Build history of the part. All positions in model axes, mm. A direction names the side the tool comes from. Give positions to 0.01 mm unless a question says otherwise; leave off trailing zeros. Write each loop counter-clockwise with the first axis right and the second up, starting at its lowest first coordinate (ties: lowest second). Pieces come first, ordered by that corner, then holes. Notation, with made-up numbers: (-9.75, 64) - (28.25, 64) arc R33 ccw to (28.25, 93) - close; hole circle Ø11 at (-37.75, 0.25). An arc over 180 degrees is marked (long way). Use one line per item in the form item = value. Start each with the question number.
from build123d import *

# Parameters (mm, degrees)
F1_DEPTH = 20
F2_W     = 5
F2_H     = 10
F3_DEPTH = 29.868809509


with BuildPart() as f1:
    # F0 (on Top) → F1 (new body)
    with BuildSketch(Plane.XY):
        with BuildLine():
            ThreePointArc((-34.9428019347, -9.9991262455), (-27.7864355102, -7.117650768), (-24.8106114437, 0))
            ThreePointArc((-24.8106114437, 0), (-27.6929606757, 7.0241759335), (-34.6784209527, 9.9991262455))
            Line((-34.6784209527, 9.9991262455), (-34.9428019347, 9.9991262455))
            Line((-34.9428019347, 9.9991262455), (-34.9428019347, 4.998252262))
            ThreePointArc((-34.9428019347, 4.998252262), (-31.3221269916, 3.581965414), (-29.8106114437, 0))
            ThreePointArc((-29.8106114437, 0), (-31.3221269916, -3.581965414), (-34.9428019347, -4.998252262))
            Line((-34.9428019347, -4.998252262), (-34.9428019347, -9.9991262455))
        make_face()
        with BuildLine():
            ThreePointArc((-34.6784209527, 9.9991262455), (-27.6929606757, 7.0241759335), (-24.8106114437, 0))
            ThreePointArc((-24.8106114437, 0), (-27.7864355102, -7.117650768), (-34.9428019347, -9.9991262455))
            Line((-34.9428019347, -9.9991262455), (-34.9428019347, -10.0008737545))
            Line((-34.9428019347, -10.0008737545), (-14.9428019347, -10.0008737545))
            Line((-14.9428019347, -10.0008737545), (-14.9428019347, 9.9991262455))
            Line((-14.9428019347, 9.9991262455), (-34.6784209527, 9.9991262455))
        make_face()
        with BuildLine():
            Line((-34.9428019347, 9.9991262455), (-34.6784209527, 9.9991262455))
            ThreePointArc((-34.6784209527, 9.9991262455), (-34.8106114437, 10), (-34.9428019347, 9.9991262455))
        make_face()
        with BuildLine():
            ThreePointArc((-34.9428019347, 9.9991262455), (-44.8106114437, 0), (-34.9428019347, -9.9991262455))
            Line((-34.9428019347, -9.9991262455), (-34.9428019347, -4.998252262))
            ThreePointArc((-34.9428019347, -4.998252262), (-39.8106114437, 0), (-34.9428019347, 4.998252262))
            Line((-34.9428019347, 4.998252262), (-34.9428019347, 9.9991262455))
        make_face()
    extrude(amount=F1_DEPTH)

    # F2 (on face) → F3 (cut, through all)
    with BuildSketch(Plane.YZ.offset(-14.9428019347)):
        with Locations((-0.0008737545, 15)):
            Rectangle(F2_W, F2_H)
    extrude(amount=-F3_DEPTH, mode=Mode.SUBTRACT)


solid = f1.part
(1) Which spindle directions (+Z, -Z, +X, -X, +Y, -Y) get a long thin tool onto all of the face, cutting with end or side? Do faces 4 (the flat face through (-27, 6, 20)), 5 (the flat face through (-23, -2.501, 15)). Say none if no direction does.
(2) Two-plate mould, pull along Y, no slides. Class faces 1 (the flat face through (-27, 0, 0)), 2 (the flat face through (-25, 9.999, 10)), 3 (the flat face through (-42, 2.499, 15)): +Y half, -Y half, draft (parallel to the pull), parting line (faces both ways), or undercut.
(3) Wall check: line 1 (Y direction, x = -22.5, z = 12); line 2 (Y direction, x = -31.5, z = 12.5); line 3 (X direction, y = -3.5, z = 19). Give the ranges that are in metal, low to high. Write a range as from..to.
(4) Cut at C-C, the plane y = -2. Give the cut face in (x, z).
(5) Cut at B-B, the plane x = -29.25. Give the cut face in (y, z).
(6) Pin check, flat tips, straight feed: pin 1 Ø10 at (y, z) = (3.5, 14) entering from -X; pin 2 Ø1.6 at (x, z) = (-42.5, 13.5) entering from +Y; pin 3 Ø5 at (y, z) = (0.5, 14.5) entering from -X. Stop position of each tip, or through.
(7) Cut at D-D, the plane y = 1. Give the cut face in (x, z), then the cut area to 3 significant figures.
Solution:
q1.face_4 = +Z, +X, -X, +Y, -Y
q1.face_5 = +Z, +X, -X
q2.face_1 = draft
q2.face_2 = +Y half
q2.face_3 = undercut
q3.line_1 = -10..-2.5, 2.5..10
q3.line_2 = -10..-3.75, 3.75..10
q3.line_3 = -44.18..-38.38, -31.24..-14.94
q4.outline = (-44.61, 0) - (-39.39, 0) - (-39.39, 10) - (-44.61, 10) - close; (-30.23, 0) - (-14.94, 0) - (-14.94, 10) - (-30.23, 10) - close
q5.outline = (-10, 0) - (10, 0) - (10, 20) - (2.5, 20) - (2.5, 10) - (-2.5, 10) - (-2.5, 20) - (-10, 20) - close
q6.pin_1 = -44.8
q6.pin_2 = 7.25
q6.pin_3 = -44.49
q7.outline = (-44.76, 0) - (-39.71, 0) - (-39.71, 10) - (-44.76, 10) - close; (-29.91, 0) - (-14.94, 0) - (-14.94, 10) - (-29.91, 10) - close
q7.area = 200 mm2
